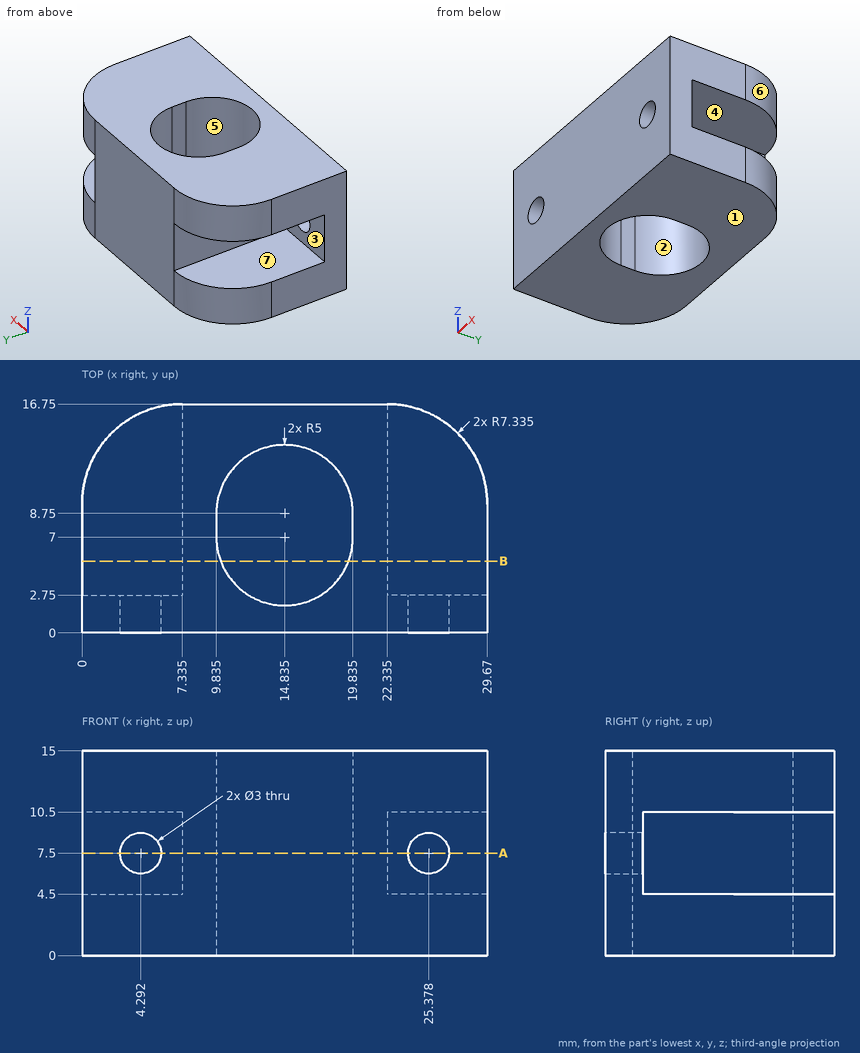
Geometry: see drawing. Coordinates: mm, zero at the bounding-box minimum. A direction names the side the tool comes from. Coordinates: 2 decimals unless noted, no trailing zeros. Loops run counter-clockwise (first coordinate to the right, second up) from the corner with the lowest first, then second, coordinate; pieces in that order, holes last. Notation, with made-up numbers: (-15, 81) -> (32, 81) arc R23 cw to (32, 114) -> close; hole circle Ø5 at (74.25, -12). An arc over 180 degrees is marked (long way). Use a Markdown table: item, result.
1) Contact query for flat-ended pins moving along their axis: pin 1 (1.8 mm diameter, centred on y = 9, z = 8, fed in from -X) (1 decimal); pin 2 (10 mm diameter, centred on x = 12, y = 11.5, fed in from -Z); pin 3 (1.4 mm diameter, centred on y = 8, z = 7, fed in from +X) (1 decimal); pin 4 (3.5 mm diameter, centred on x = 4.29, z = 7.5, fed in from +Y). Output: stop coordinate, or through.
Results found:
| item | result |
|---|---|
| pin 1 | stops at x = 7.3 |
| pin 2 | stops at z = 0 |
| pin 3 | stops at x = 22.3 |
| pin 4 | stops at y = 2.75 |
2) Cut plane B-B (y = 5.25). Return the cut outline in (x, z) (1 decimal).
Results found:
| item | result |
|---|---|
| outline | (0, 0) -> (10.2, 0) -> (10.2, 15) -> (0, 15) -> (0, 10.5) -> (7.3, 10.5) -> (7.3, 4.5) -> (0, 4.5) -> close; (19.5, 0) -> (29.7, 0) -> (29.7, 4.5) -> (22.3, 4.5) -> (22.3, 10.5) -> (29.7, 10.5) -> (29.7, 15) -> (19.5, 15) -> close |
3) Pull-direction query (Z, two-part tool) for the marked faces 1, 2 and 3; classes: released by +Z, released by -Z, zero draft, split by the parting line, or undercut.
Results found:
| item | result |
|---|---|
| face 1 | released by -Z |
| face 2 | zero draft |
| face 3 | undercut |
4) Material intervals for line 1 along X through (y, z) = (1.2, 7.5); line 2 along Z through (x, y) = (6.25, 13.5); line 3 along X through (y, z) = (9.25, 7.75) (1 decimal), sorted ascending. Write a range as from..to.
Results found:
| item | result |
|---|---|
| line 1 | x = 0..2.79, 5.79..23.88, 26.88..29.67 |
| line 2 | z = 0..4.5, 10.5..15 |
| line 3 | x = 7.3..9.9, 19.8..22.3 |
5) Access query for the marked faces 4, 5, 6 and 7. Directions: +Z, -Z, +X, -X, +Y, -Y. A direction counts if a zero-diameter tool reaches every point of the face in a straight line with its end or side. Return the directions, or none.
Results found:
| item | result |
|---|---|
| face 4 | +X, +Y |
| face 5 | +Z, -Z |
| face 6 | +Z, -Z, +X, +Y |
| face 7 | -X, +Y |
6) Cut plane A-A (z = 7.5). Give the number of separate pieces and of enclosed holes in the cut face, then the cut area to 3 significant figures.
Results found:
| item | result |
|---|---|
| separate pieces | 3 |
| enclosed holes | 1 |
| area | 179 mm2 |
